```python
from build123d import *

# Parameters (mm, degrees)
SALIENTE_EXTRUIR1_DEPTH = 34.5
CROQUIS2_R              = 9
CORTAR_EXTRUIR1_DEPTH   = 26
CROQUIS3_W              = 10
CROQUIS3_H              = 5
CROQUIS3_W_2            = 10.5
CROQUIS3_W_3            = 20.5
CORTAR_EXTRUIR2_DEPTH   = 3.5
CROQUIS4_R              = 3
CORTAR_EXTRUIR3_DEPTH   = 13


with BuildPart() as part:
    # Croquis1 → Saliente-Extruir1 (new body)
    with BuildSketch(Plane.XY):
        Polygon((0, 0), (0, 12), (16.5, 12), (16.5, 9), (39, 9), (39, 12), (87, 12), (87, 9), (109.5, 9), (109.5, 12), (126, 12), (126, 0), align=None)
    extrude(amount=SALIENTE_EXTRUIR1_DEPTH)

    # Croquis2 → Cortar-Extruir1 (cut)
    with BuildSketch(Plane(origin=(0, 0, 0), x_dir=(-1, 0, 0), z_dir=(0, 0, -1))):
        with Locations((-63, 12)):
            Circle(CROQUIS2_R)
    extrude(amount=-CORTAR_EXTRUIR1_DEPTH, mode=Mode.SUBTRACT)

    # Croquis3 → Cortar-Extruir2 (cut)
    with BuildSketch(Plane(origin=(0, 9, 0), x_dir=(1, 0, 0), z_dir=(0, 1, 0))):
        with Locations((22.5, -29)):
            Rectangle(CROQUIS3_W, CROQUIS3_H)
        with Locations((32.75, -29)):
            Rectangle(CROQUIS3_W_2, CROQUIS3_H)
        with Locations((32.75, -21)):
            Rectangle(CROQUIS3_W_2, CROQUIS3_H)
        with Locations((22.5, -21)):
            Rectangle(CROQUIS3_W, CROQUIS3_H)
        with Locations((32.75, -13)):
            Rectangle(CROQUIS3_W_2, CROQUIS3_H)
        with Locations((22.5, -13)):
            Rectangle(CROQUIS3_W, CROQUIS3_H)
        with Locations((32.75, -5)):
            Rectangle(CROQUIS3_W_2, CROQUIS3_H)
        with Locations((22.5, -5)):
            Rectangle(CROQUIS3_W, CROQUIS3_H)
        with Locations((98.25, -29)):
            Rectangle(CROQUIS3_W_3, CROQUIS3_H)
        with Locations((98.25, -21)):
            Rectangle(CROQUIS3_W_3, CROQUIS3_H)
        with Locations((98.25, -13)):
            Rectangle(CROQUIS3_W_3, CROQUIS3_H)
        with Locations((98.25, -5)):
            Rectangle(CROQUIS3_W_3, CROQUIS3_H)
    extrude(amount=-CORTAR_EXTRUIR2_DEPTH, mode=Mode.SUBTRACT)

    # Croquis4 → Cortar-Extruir3 (cut, through all)
    with BuildSketch(Plane(origin=(0, 12, 0), x_dir=(1, 0, 0), z_dir=(0, 1, 0))):
        with Locations((6.5, -15)):
            Circle(CROQUIS4_R)
    cortar_extruir3 = extrude(amount=-CORTAR_EXTRUIR3_DEPTH, mode=Mode.SUBTRACT)

    # Simetría1: Cortar-Extruir3 across plane
    add(cortar_extruir3.mirror(Plane.ZY.offset(-63)), mode=Mode.SUBTRACT)


solid = part.part
```
Can you work these out from the model? Positions are in its coordinate system, mm. A direction names the side the tool comes from. Round coordinates to 2 decimals unless told otherwise and drop trailing zeros. Loops run counter-clockwise (first coordinate to the right, second up) from the corner with the lowest first, then second, coordinate; pieces in that order, holes last. Notation, with made-up numbers: M 11.5,32.25 L 16.5,32.25 A20 ccw 16.5,38.25 Z; hole C 26.25,83.5 d6. An arc over 180 degrees is marked long. Answer as a JSON object with one key per item and string values. Group by question number.
Q1. Imagine slicing it at A-A, the plane x = 6.5. Please give me the cut outline in (y, z), then the cut area to 3 significant figures.
Q2. Imagine slicing it at D-D, the plane x = 92. Please give me the cut outline in (y, z), then the cut area to 4 significant figures.
Q3. Will this pin go through, and if not, where does the flat tip stop? pin 1 (5.5 mm diameter, centred on x = 31.5, z = 29.5, fed in from +Y).
Q4. We'd pull the mould along Z, two halves only. Please class faces 1 (the flat face through (64, 2, 0)), 2 (the flat face through (28, 9, 17)), 3 (the flat face through (98, 5.5, 29)): +Z half, -Z half, draft (parallel to the pull), parting line (faces both ways), or undercut.
Q5. Please list where these lines run through material, in increasing order: L1, parallel to X at y = 8, z = 28; L2, parallel to Z at x = 6.5, y = 8.75; L3, parallel to Z at x = 105, y = 8.5.
Q6. Imagine slicing it at B-B, the plane z = 21.5. Please give me the cut outline in (x, y).
Q7. Imagine slicing it at C-C, the plane x = 63. Please give me the cut outline in (y, z).
Q8. On a 3-axis mill with a long thin cutter (end or side, diameter ignored), from which of +Z, -Z, +X, -X, +Y, -Y can I reach the whole of each face in a straight line? I mean faces 4 (the cylindrical face through (7.884, 6.084, 17.662)), 5 (the flat face through (39, 10, 17)), 6 (the flat face through (98, 7, 2.5)). Say none if no direction works.
Findings:
{
 "1": {"outline": "M 0,0 L 12,0 L 12,12 L 0,12 Z; M 0,18 L 12,18 L 12,34.5 L 0,34.5 Z", "area": "342 mm2"},
 "2": {"outline": "M 0,0 L 9,0 L 9,2.5 L 5.5,2.5 L 5.5,7.5 L 9,7.5 L 9,10.5 L 5.5,10.5 L 5.5,15.5 L 9,15.5 L 9,18.5 L 5.5,18.5 L 5.5,23.5 L 9,23.5 L 9,26.5 L 5.5,26.5 L 5.5,31.5 L 9,31.5 L 9,34.5 L 0,34.5 Z", "area": "240.5 mm2"},
 "3": {"pin 1": "stops at y = 9"},
 "4": {"face 1": "-Z half", "face 2": "draft", "face 3": "undercut"},
 "5": {"L1": "x = 0 to 17.5, 38 to 88, 108.5 to 126", "L2": "z = 0 to 12, 18 to 34.5", "L3": "z = 0 to 2.5, 7.5 to 10.5, 15.5 to 18.5, 23.5 to 26.5, 31.5 to 34.5"},
 "6": {"outline": "M 0,0 L 126,0 L 126,12 L 109.5,12 L 109.5,9 L 108.5,9 L 108.5,5.5 L 88,5.5 L 88,9 L 87,9 L 87,12 L 72,12 A9 cw 54,12 L 39,12 L 39,9 L 38,9 L 38,5.5 L 17.5,5.5 L 17.5,9 L 16.5,9 L 16.5,12 L 0,12 Z"},
 "7": {"outline": "M 0,0 L 3,0 L 3,26 L 12,26 L 12,34.5 L 0,34.5 Z"},
 "8": {"face 4": "+Y, -Y", "face 5": "+Z, -Z, +Y", "face 6": "+Y"}
}
